Geometry: final body of the model. Coordinates: model frame, mm. A direction names the side the tool comes from. Give positions to 0.01 mm unless a question says otherwise; leave off trailing zeros. Order: outer loops, then holes, each group sorted by start corner. A loop starts at its lowest first (then second) coordinate and runs counter-clockwise, first axis right, second up. Notation, with made-up numbers: (-18.5, -24.75) - (37.5, -24.75) arc R12 ccw to (37.5, -1.75) - close; hole circle Ø9 at (-2, -33). An arc over 180 degrees is marked (long way). One line per item, written item: value.
Autodesk Inventor part; units mm, degrees
ref_plane "YZ Plane" through (0, 0, 0) normal (1, 0, 0) x (0, 1, 0)
ref_plane "XZ Plane" through (0, 0, 0) normal (0, 1, 0) x (-1, 0, 0)
ref_plane "XY Plane" through (0, 0, 0) normal (0, 0, 1) x (1, 0, 0)
sketch "Sketch1" plane through (0, 0, 0) normal (0, 0, 1) x (1, 0, 0)
  circle A0 centre (0, 0) radius 21.1
  circle A1 centre (0, 0) radius 22
  circle A2 centre (0, 0) radius 12.8
  circle A3 centre (0, 0) radius 11.7
  circle A4 centre (0, 22) radius 0.5
  dimension "d1" = 44
  dimension "d0" = 42.2
  dimension "d2" = 25.6
  dimension "d3" = 23.4
  dimension "d13" = 1
extrude "Extrusion1" add sketch "Sketch1" against normal blind 4 contours A0
extrude "Extrusion2" add sketch "Sketch1" against normal blind 20 contours A1 A4 | A4 A1 picked at (5.1126, 20.6747) picked at (0.0199, 21.8341)
extrude "Extrusion3" add sketch "Sketch1" against normal blind 1 contours A2
chamfer "Chamfer1" distance 2 angle 45 1 edges at (-22, 0, 0)
sketch "Sketch2" plane through (0, 0, -20) normal (0, 0, -1) x (-1, 0, 0)
  circle A0 centre (0, 0) radius 22
  line L0 (0.5, 21) -> (-0.5, 21)
  line L1 (-0.5, 21) -> (-0.5, 23)
  line L2 (-0.5, 23) -> (0.5, 23)
  line L3 (0.5, 23) -> (0.5, 21)
  line L4 (0.5, 21) -> (-0.5, 23) construction
  line L5 (-0.5, 21) -> (0.5, 23) construction
  point P0 (0, 22)
  dimension "d15" = 1
  dimension "d16" = 2
extrude "Extrusion4" cut sketch "Sketch2" against normal blind 20 contours L3 L0 L1 A0 | A0 L1 L2 L3 picked at (-0.0556, 21.3331)
properties part number "PolarizerObjectiveCap-MitutoyoPlanApoBD"
1) Section A-A, the plane z = -4.75. Return loops of the section in (x, y), then the cut area to 3 significant figures.
Answers below:
outline: (-0.5, 21.09) - (-0.5, 21.99) arc R22 ccw (long way) to (0.5, 21.99) - (0.5, 21.09) arc R21.1 cw (long way) to start
area: 121 mm^2
2) First-contact query: pin 1 (3 mm diameter, centred on x = -15, y = 13.5, fed in from -Z); pin 2 (5 mm diameter, centred on x = 12.5, y = 6.5, fed in from -Z); pin 3 (4 mm diameter, centred on y = -8, z = -9, fed in from -X); pin 4 (2 mm diameter, centred on x = -8.5, y = -2, fed in from +Z). Flat tips, straight axial feed; report the tip coordinate or a pass-through.
Answers below:
pin 1: z = -20
pin 2: z = -4
pin 3: x = -21.17
pin 4: through
3) Material intervals for line 1 along Y through (x, z) = (0, -2.65); line 2 along Z through (x, y) = (17.5, 0.5); line 3 along X through (y, z) = (10, -17.25), sorted ascending.
Answers below:
line 1: -22 to -12.8, 12.8 to 21
line 2: -4 to 0
line 3: -19.6 to -18.58, 18.58 to 19.6
4) Mould query, pull axis X, two halves, no side actions, for faces 4 (the face through (-2.54, -11.42, -0.49)), 5 (the face through (-4.36, 19.65, -0.13)), 6 (the face through (-21.3, 0.1, -20)). Classes: released by +X, released by -X, zero draft, split by the parting line, or undercut.
Answers below:
face 4: undercut
face 5: split by the parting line
face 6: zero draft
5) Set-up query: faces 1 (the face through (0, 21, -3)), 2 (the face through (-10.158, -7.789, -2.479)), 3 (the face through (9, -9, 0)). Return all of +Z, -Z, +X, -X, +Y, -Y with unobstructed straight access to the full face (end or side cutting, diameter ignored); none if empty.
Answers below:
face 1: +Z, -Z, +Y
face 2: -Z
face 3: +Z, +X, -X, +Y, -Y
